from build123d import *

# Parameters (mm, degrees)
PAD_DEPTH       = 300
SKETCH001_R     = 2.2
POCKET_DEPTH    = 14.588933
SKETCH002_R     = 3.7
POCKET001_DEPTH = 5


with BuildPart() as part:
    # Sketch → Pad (new body)
    with BuildSketch(Plane.XY):
        with BuildLine():
            Line((-7, 0), (7, 0))
            ThreePointArc((7, 0), (7.428584, 0.242481), (7.441474, 0.734736))
            Line((3, 9.087933), (7.441474, 0.734736))
            Line((7.364852, 13.746052), (3, 9.087933))
            ThreePointArc((7.364852, 13.746052), (7.458771, 14.286754), (7, 14.587933))
            Line((7, 14.587933), (-7, 14.587933))
            ThreePointArc((-7, 14.587933), (-7.458771, 14.286754), (-7.364852, 13.746052))
            Line((-7.364852, 13.746052), (-3, 9.087933))
            Line((-3, 9.087933), (-7.441474, 0.734736))
            ThreePointArc((-7.441474, 0.734736), (-7.428584, 0.242481), (-7, 0))
        make_face()
    extrude(amount=PAD_DEPTH)

    # Sketch001 (on Face2 of Pad) → Pocket (cut, through all)
    with BuildSketch(Plane(origin=(0, 14.587933, 0), x_dir=(-1, 0, 0), z_dir=(0, 1, 0))):
        with Locations((0, 20)):
            Circle(SKETCH001_R)
        with Locations((0, 80)):
            Circle(SKETCH001_R)
        with Locations((0, 140)):
            Circle(SKETCH001_R)
        with Locations((0, 200)):
            Circle(SKETCH001_R)
        with Locations((0, 260)):
            Circle(SKETCH001_R)
    extrude(amount=-POCKET_DEPTH, mode=Mode.SUBTRACT)

    # Sketch002 → Pocket001 (cut)
    with BuildSketch(Plane(origin=(0, 14.587933, 0), x_dir=(-1, 0, 0), z_dir=(0, 1, 0))):
        with Locations((0, 260)):
            Circle(SKETCH002_R)
        with Locations((0, 200)):
            Circle(SKETCH002_R)
        with Locations((0, 140)):
            Circle(SKETCH002_R)
        with Locations((0, 80)):
            Circle(SKETCH002_R)
        with Locations((0, 20)):
            Circle(SKETCH002_R)
    extrude(amount=-POCKET001_DEPTH, mode=Mode.SUBTRACT)


solid = part.part
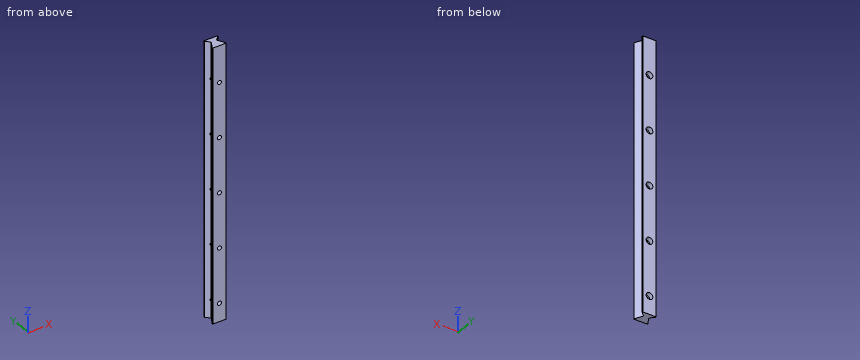
Could you check a few things on this model? Use its own coordinates, in mm. Give positions to 0.01 mm unless a question says otherwise; leave off trailing zeros. Order: outer loops, then holes, each group sorted by start corner. A loop starts at its lowest first (then second) coordinate and runs counter-clockwise, first axis right, second up. Notation, with made-up numbers: (-36.5, -1) - (8.5, -1) arc R21 ccw to (8.5, 8) - close; hole circle Ø9 at (9.25, 24.5). An arc over 180 degrees is marked (long way). One line per item, written item: value. Start each with the question number.
1. For P1, Ø8, axis at y = 8, z = 60, coming from the +X side; P2, Ø5.5, axis at x = 0, z = 200, coming from the +Y side; P3, Ø1.5, axis at y = 1.5, z = 76.5, coming from the -X side; P4, Ø2, axis at x = -1, z = 139.5, coming from the +Y side, each with a flat end and sliding along its axis, tell me the tip position at first contact or that it passes through.
2. Imagine slicing it at B-B on y = 3. List the corners of the cut face in (x, z) for me, plus the area to 3 significant figures.
3. Imagine slicing it at A-A on z = 223. List the corners of the cut face in (x, y) for me, plus the area to 3 significant figures.
4. If I drill on probe 1 along Z at (x, y) = (0, 12.5); probe 2 along Z at (x, y) = (0, 6.25); probe 3 along X at (y, z) = (13.3, 20), over which ranges is the centre line in solid material (lowest first)?
Values:
1. P1: x = 5.73
1. P2: y = 9.59
1. P3: x = -7.43
1. P4: through
2. outline: (-6.24, 0) - (6.24, 0) - (6.24, 300) - (-6.24, 300) - close; hole circle Ø4.4 at (0, 20); hole circle Ø4.4 at (0, 80); hole circle Ø4.4 at (0, 140); hole circle Ø4.4 at (0, 200); hole circle Ø4.4 at (0, 260)
2. area: 3,670 mm²
3. outline: (-7.44, 0.73) arc R0.5 ccw to (-7, 0) - (7, 0) arc R0.5 ccw to (7.44, 0.73) - (3, 9.09) - (7.36, 13.75) arc R0.5 ccw to (7, 14.59) - (-7, 14.59) arc R0.5 ccw to (-7.36, 13.75) - (-3, 9.09) - close
3. area: 159 mm²
4. probe 1: 0 to 16.3, 23.7 to 76.3, 83.7 to 136.3, 143.7 to 196.3, 203.7 to 256.3, 263.7 to 300
4. probe 2: 0 to 17.8, 22.2 to 77.8, 82.2 to 137.8, 142.2 to 197.8, 202.2 to 257.8, 262.2 to 300
4. probe 3: -6.95 to -3.7, 3.7 to 6.95
